Print and shaded views of the part. All mm, measured from the part's lowest x, y and z. Give positions to 0.01 mm unless a question says otherwise; leave off trailing zeros. Loops run counter-clockwise (first coordinate to the right, second up) from the corner with the lowest first, then second, coordinate; pieces in that order, holes last. Notation, with made-up numbers: (29, 72) - (59, 72) arc R22 cw to (59, 111) - close; hole circle Ø4 at (-4, -23). An arc over 180 degrees is marked (long way). Return JSON: item names as keys, results as strings.
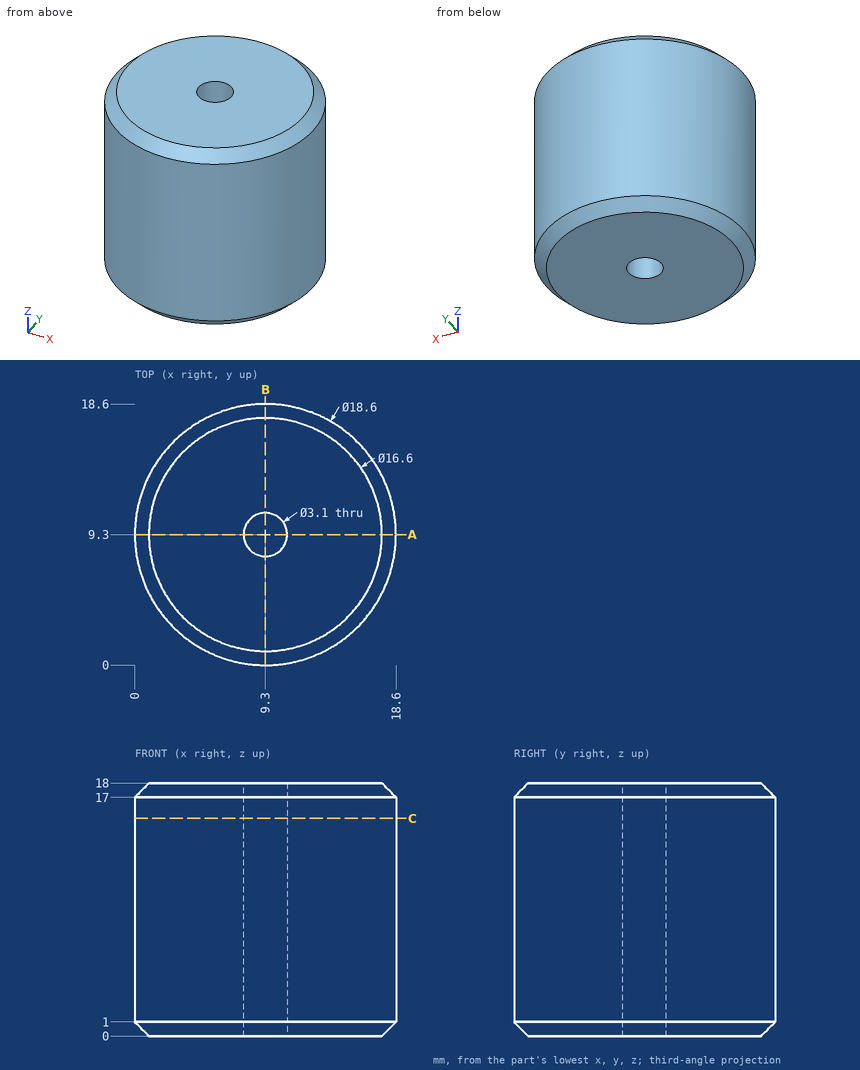
1. Drill centre lines: probe 1 along Y at (x, z) = (9.3, 5.5); probe 2 along X at (y, z) = (9, 7); probe 3 along X at (y, z) = (1.75, 6.75). Where is each one in solid material? Low to high.
Values follow:
{"probe 1": "y = 0 to 7.75, 10.85 to 18.6", "probe 2": "x = 0 to 7.78, 10.82 to 18.6", "probe 3": "x = 3.87 to 14.73"}
2. Cut at C-C, the plane z = 15.5. Write the cut outline in (x, y).
Values follow:
{"outline": "circle Ø18.6 at (9.3, 9.3); hole circle Ø3.1 at (9.3, 9.3)"}
3. Cut at A-A, the plane y = 9.3. Write the cut outline in (x, z), plus the area to 3 significant figures.
Values follow:
{"outline": "(0, 1) - (1, 0) - (7.75, 0) - (7.75, 18) - (1, 18) - (0, 17) - close; (10.85, 0) - (17.6, 0) - (18.6, 1) - (18.6, 17) - (17.6, 18) - (10.85, 18) - close", "area": "277 mm²"}
4. Drop flat-ended pins along their axis: P1, Ø10, axis at x = 2.5, z = 8.5, coming from the +Y side; P2, Ø8, axis at y = 14.5, z = 15, coming from the +X side; P3, Ø8, axis at x = 14.5, z = 13.5, coming from the +Y side. Give the stop position or say it passes through.
Values follow:
{"P1": "stops at y = 18.42", "P2": "stops at x = 18.52", "P3": "stops at y = 18.52"}
